Can you work these out from the model? Positions are in its coordinate system, mm. A direction names the side the tool comes from. Coordinates: 2 decimals unless noted, no trailing zeros. Order: outer loops, then holes, each group sorted by start corner. A loop starts at its lowest first (then second) coordinate and runs counter-clockwise, first axis right, second up. Notation, with made-up numbers: (-23.75, 40.5) - (-2.75, 40.5) arc R22 cw to (-2.75, 69.5) - close; hole circle Ø8 at (33.25, 30). An arc over 180 degrees is marked (long way). Use a Markdown table: item, result. Add a question column.
(1) On a 3-axis mill with a long thin cutter (end or side, diameter ignored), from which of +Z, -Z, +X, -X, +Y, -Y can I reach the whole of each face in a straight line? I mean faces 4 (the flat face through (-40.3, -3.1, 5.5)), 5 (the flat face through (0, -35, 3)), 6 (the flat face through (-36, 0, 1)), 7 (the flat face through (-44, 0, 3.5)), 8 (the flat face through (-36, 0, 4.5)). Say none if no direction works.
(2) I want a section at C-C (x = 42.5). List the corners of the cut face in (y, z) for me.
(3) For pin 1 Ø8 at (x, y) = (34.5, 17) entering from +Z; pin 2 Ø3 at (x, y) = (12.5, -33) entering from +Z, each with a flat end and sliding along its axis, tell me the tip position at first contact or that it passes through.
(4) If I drill on L1, parallel to Y at x = -3, z = 4.25; L2, parallel to X at y = 3.5, z = 1.8; L3, parallel to Y at x = -30, z = 4.65, over which ranges is the centre line in solid material (lowest first)? Write a range as [from, to].
(5) I want a section at A-A (y = 6.5). State how many separate pieces and enclosed holes the cut face has, and give its area (3 significant figures).
(6) We'd pull the mould along X, two halves only. Please class faces 1 (the flat face through (60, -1, 3)), 2 (the flat face through (-55, 0, 3)), 3 (the flat face through (-40.3, -3.1, 0)): pulls with the +X half, pulls with the -X half, needs draft (parallel to the pull), parting line crosses it, or undercut.
(7) I want a section at B-B (x = -11). List the corners of the cut face in (y, z) for me, and give its area (3 significant figures).
```python
from build123d import *

# Parameters (mm, degrees)
F0_W     = 120
F0_H     = 90
F0_W_2   = 5
F0_H_2   = 10
F1_DEPTH = 2
F2_START = 2
F2_DEPTH = 1.5
F3_START = 3.5
F3_DEPTH = 2
F4_START = 1
F4_DEPTH = 1
F5_START = 2
F5_DEPTH = 1.5
F6_START = 3.5
F6_DEPTH = 1


with BuildPart() as f1:
    # F0 (on Top) → F1 (new body)
    with BuildSketch(Plane.XY):
        Rectangle(F0_W, F0_H)
        Polygon((40, 40), (40, 25), (50, 25), (50, 10), (55, 10), (55, -10), (50, -10), (50, -25), (40, -25), (40, -40), (-40, -40), (-40, -25), (-50, -25), (-50, -10), (-55, -10), (-55, 10), (-50, 10), (-50, 25), (-40, 25), (-40, 40), align=None, mode=Mode.SUBTRACT)
        Polygon((-40, 15), (-40, 25), (-50, 25), (-50, 10), (-50, -10), (-50, -25), (-40, -25), (-40, -15), (-45, -15), (-45, -5), (-40, -5), (-40, 5), (-45, 5), (-45, 15), align=None)
        Polygon((50, 25), (40, 25), (40, 15), (45, 15), (45, 5), (40, 5), (40, -5), (45, -5), (45, -15), (40, -15), (40, -25), (50, -25), (50, -10), (50, 10), align=None)
        with Locations((42.5, 10)):
            Rectangle(F0_W_2, F0_H_2)
        with Locations((42.5, -10)):
            Rectangle(F0_W_2, F0_H_2)
        with Locations((-42.5, -10)):
            Rectangle(F0_W_2, F0_H_2)
        with Locations((-42.5, 10)):
            Rectangle(F0_W_2, F0_H_2)
    extrude(amount=F1_DEPTH)

    # F0 (on Top) → F2 (join)
    with BuildSketch(Plane.XY.offset(F2_START)):
        Rectangle(F0_W, F0_H)
        Polygon((40, 40), (40, 25), (50, 25), (50, 10), (55, 10), (55, -10), (50, -10), (50, -25), (40, -25), (40, -40), (-40, -40), (-40, -25), (-50, -25), (-50, -10), (-55, -10), (-55, 10), (-50, 10), (-50, 25), (-40, 25), (-40, 40), align=None, mode=Mode.SUBTRACT)
        with Locations((-42.5, -10)):
            Rectangle(F0_W_2, F0_H_2)
        with Locations((-42.5, 10)):
            Rectangle(F0_W_2, F0_H_2)
        with Locations((42.5, 10)):
            Rectangle(F0_W_2, F0_H_2)
        with Locations((42.5, -10)):
            Rectangle(F0_W_2, F0_H_2)
    extrude(amount=F2_DEPTH)

    # F0 (on Top) → F3 (join)
    with BuildSketch(Plane.XY.offset(F3_START)):
        Rectangle(F0_W, F0_H)
        Polygon((40, 40), (40, 25), (50, 25), (50, 10), (55, 10), (55, -10), (50, -10), (50, -25), (40, -25), (40, -40), (-40, -40), (-40, -25), (-50, -25), (-50, -10), (-55, -10), (-55, 10), (-50, 10), (-50, 25), (-40, 25), (-40, 40), align=None, mode=Mode.SUBTRACT)
        Polygon((-40, 15), (-40, 25), (-50, 25), (-50, 10), (-50, -10), (-50, -25), (-40, -25), (-40, -15), (-45, -15), (-45, -5), (-40, -5), (-40, 5), (-45, 5), (-45, 15), align=None)
        Polygon((50, 25), (40, 25), (40, 15), (45, 15), (45, 5), (40, 5), (40, -5), (45, -5), (45, -15), (40, -15), (40, -25), (50, -25), (50, -10), (50, 10), align=None)
        with Locations((42.5, 10)):
            Rectangle(F0_W_2, F0_H_2)
        with Locations((42.5, -10)):
            Rectangle(F0_W_2, F0_H_2)
        with Locations((-42.5, -10)):
            Rectangle(F0_W_2, F0_H_2)
        with Locations((-42.5, 10)):
            Rectangle(F0_W_2, F0_H_2)
    extrude(amount=F3_DEPTH)

    # F0 (on Top) → F4 (join)
    with BuildSketch(Plane.XY.offset(F4_START)):
        Polygon((40, -25), (35, -25), (35, -35), (-35, -35), (-35, -25), (-40, -25), (-40, -40), (40, -40), align=None)
        with Locations((-37.5, -20)):
            Rectangle(F0_W_2, F0_H_2)
        with Locations((-37.5, -10)):
            Rectangle(F0_W_2, F0_H_2)
        with Locations((-37.5, 0)):
            Rectangle(F0_W_2, F0_H_2)
        with Locations((-37.5, 10)):
            Rectangle(F0_W_2, F0_H_2)
        with Locations((-37.5, 20)):
            Rectangle(F0_W_2, F0_H_2)
        Polygon((-35, 35), (35, 35), (35, 25), (40, 25), (40, 40), (-40, 40), (-40, 25), (-35, 25), align=None)
        with Locations((37.5, 20)):
            Rectangle(F0_W_2, F0_H_2)
        with Locations((37.5, 10)):
            Rectangle(F0_W_2, F0_H_2)
        with Locations((37.5, 0)):
            Rectangle(F0_W_2, F0_H_2)
        with Locations((37.5, -10)):
            Rectangle(F0_W_2, F0_H_2)
        with Locations((37.5, -20)):
            Rectangle(F0_W_2, F0_H_2)
    extrude(amount=F4_DEPTH)

    # F0 (on Top) → F5 (join)
    with BuildSketch(Plane.XY.offset(F5_START)):
        with Locations((-37.5, 10)):
            Rectangle(F0_W_2, F0_H_2)
        with Locations((-37.5, -10)):
            Rectangle(F0_W_2, F0_H_2)
        Polygon((40, -25), (35, -25), (35, -35), (-35, -35), (-35, -25), (-40, -25), (-40, -40), (40, -40), align=None)
        with Locations((37.5, -10)):
            Rectangle(F0_W_2, F0_H_2)
        with Locations((37.5, 10)):
            Rectangle(F0_W_2, F0_H_2)
        Polygon((-35, 35), (35, 35), (35, 25), (40, 25), (40, 40), (-40, 40), (-40, 25), (-35, 25), align=None)
    extrude(amount=F5_DEPTH)

    # F0 (on Top) → F6 (join)
    with BuildSketch(Plane.XY.offset(F6_START)):
        Polygon((-35, 35), (35, 35), (35, 25), (40, 25), (40, 40), (-40, 40), (-40, 25), (-35, 25), align=None)
        with Locations((-37.5, 20)):
            Rectangle(F0_W_2, F0_H_2)
        with Locations((-37.5, 10)):
            Rectangle(F0_W_2, F0_H_2)
        with Locations((-37.5, 0)):
            Rectangle(F0_W_2, F0_H_2)
        with Locations((-37.5, -10)):
            Rectangle(F0_W_2, F0_H_2)
        with Locations((-37.5, -20)):
            Rectangle(F0_W_2, F0_H_2)
        Polygon((40, -25), (35, -25), (35, -35), (-35, -35), (-35, -25), (-40, -25), (-40, -40), (40, -40), align=None)
        with Locations((37.5, -20)):
            Rectangle(F0_W_2, F0_H_2)
        with Locations((37.5, -10)):
            Rectangle(F0_W_2, F0_H_2)
        with Locations((37.5, 0)):
            Rectangle(F0_W_2, F0_H_2)
        with Locations((37.5, 10)):
            Rectangle(F0_W_2, F0_H_2)
        with Locations((37.5, 20)):
            Rectangle(F0_W_2, F0_H_2)
    extrude(amount=F6_DEPTH)


solid = f1.part
```
Answers follow:
| question | item | result |
|---|---|---|
| 1 | face 4 | +Z, +X, -X, +Y, -Y |
| 1 | face 5 | +Z, -Z |
| 1 | face 6 | -Z |
| 1 | face 7 | none |
| 1 | face 8 | +Z |
| 2 | outline | (-45, 0) - (45, 0) - (45, 5.5) - (-45, 5.5) - close; hole (-25, 2) - (-15, 2) - (-15, 3.5) - (-25, 3.5) - close; hole (-5, 2) - (5, 2) - (5, 3.5) - (-5, 3.5) - close; hole (15, 2) - (25, 2) - (25, 3.5) - (15, 3.5) - close |
| 3 | pin 1 | stops at z = 4.5 |
| 3 | pin 2 | passes through |
| 4 | L1 | y = [-45, -35], [35, 45] |
| 4 | L2 | x = [-60, -55], [-50, -35], [35, 50], [55, 60] |
| 4 | L3 | y = [-45, -40], [40, 45] |
| 5 | separate pieces | 4 |
| 5 | enclosed holes | 0 |
| 5 | area | 185 mm² |
| 6 | face 1 | pulls with the +X half |
| 6 | face 2 | undercut |
| 6 | face 3 | needs draft |
| 7 | outline | (-45, 0) - (-40, 0) - (-40, 1) - (-35, 1) - (-35, 4.5) - (-40, 4.5) - (-40, 5.5) - (-45, 5.5) - close; (35, 1) - (40, 1) - (40, 0) - (45, 0) - (45, 5.5) - (40, 5.5) - (40, 4.5) - (35, 4.5) - close |
| 7 | area | 90.0 mm² |
